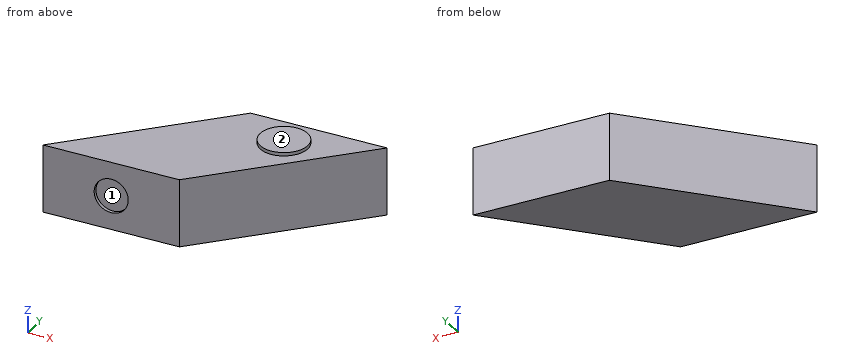
from build123d import *

# Parameters (mm, degrees)
BOSS_EXTRU_1_DEPTH      = 200
ESQUISSE2_R             = 70
BOSS_EXTRU_2_DEPTH      = 10
ESQUISSE3_R             = 50
ENL_V_MAT_EXTRU_1_DEPTH = 10


with BuildPart() as part:
    # Esquisse1 → Boss.-Extru.1 (new body)
    with BuildSketch(Plane.XY):
        Polygon((0, 0), (400, 400), (800, 400), (400, 0), align=None)
    extrude(amount=BOSS_EXTRU_1_DEPTH)

    # Esquisse2 → Boss.-Extru.2 (add)
    with BuildSketch(Plane.XY.offset(200)):
        with Locations((550, 300)):
            Circle(ESQUISSE2_R)
    extrude(amount=BOSS_EXTRU_2_DEPTH)

    # Esquisse3 → Enlèv. mat.-Extru.1 (cut)
    with BuildSketch(Plane(origin=(0, 0, 0), x_dir=(-1, 0, 0), z_dir=(0, -1, 0))):
        with Locations(Location((-200, -100, 0), (0, 0, 90))):
            Circle(ESQUISSE3_R)
    extrude(amount=-ENL_V_MAT_EXTRU_1_DEPTH, mode=Mode.SUBTRACT)


solid = part.part
Verification items for the finished model (mm, model axes). Face numbers are marked on the shaded views. A direction names the side the tool comes from. Give positions to 0.01 mm unless a question says otherwise; leave off trailing zeros. Loops run counter-clockwise (first coordinate to the right, second up) from the corner with the lowest first, then second, coordinate; pieces in that order, holes last.
1. Cross-section at A-A on y = 258. Record the cut outline in (x, z), and give its area (3 significant figures).
Derived:
outline: (258, 0) - (658, 0) - (658, 200) - (606, 200) - (606, 210) - (494, 210) - (494, 200) - (258, 200) - close
area: 81,100 mm2
2. Cross-section at C-C on x = 414. Record the cut outline in (y, z).
Derived:
outline: (14, 0) - (400, 0) - (400, 200) - (14, 200) - close
3. Go/stop test with flat-tipped pins: P1, Ø2, axis at y = 251, z = 55.5, coming from the +X side; P2, Ø8, axis at y = 267, z = 23.5, coming from the +X side; P3, Ø5, axis at y = 290.5, z = 154.5, coming from the +X side. Record where each tip stops, or that it passes through.
Derived:
P1: stops at x = 652
P2: stops at x = 671
P3: stops at x = 693
4. Cross-section at D-D on z = 168.5. Record the cut outline in (x, y).
Derived:
outline: (0, 0) - (400, 0) - (800, 400) - (400, 400) - close
5. Material ranges on probe 1 along Z at (x, y) = (417, 342.5); probe 2 along X at (y, z) = (2, 100); probe 3 along X at (y, z) = (6.25, 100), recorded low to high.
Derived:
probe 1: z = 0 to 200
probe 2: x = 2 to 150, 250 to 402
probe 3: x = 6.25 to 150, 250 to 406.25
6. Cross-section at B-B on z = 100. Record the cut outline in (x, y), and give its area (3 significant figures).
Derived:
outline: (0, 0) - (150, 0) - (150, 10) - (250, 10) - (250, 0) - (400, 0) - (800, 400) - (400, 400) - close
area: 159,000 mm2
7. Tool access check on the marked faces 1 and 2. Record the directions out of +Z, -Z, +X, -X, +Y, -Y that give a thin tool (end or side, any length) a straight path to the whole face; none if there is none.
Derived:
face 1: -Y
face 2: +Z, +X, -X, +Y, -Y
